Could you check a few things on this model? Use its own coordinates, in mm. Face numbers are marked on the shaded views. Coordinates: 2 decimals unless noted, no trailing zeros. Write each loop counter-clockwise with the first axis right and the second up, starting at its lowest first coordinate (ties: lowest second). Pieces come first, ordered by that corner, then holes. Notation, with made-up numbers: (10.5, 62.5) - (54.5, 62.5) arc R19 cw to (54.5, 69.5) - close; hole circle Ø4 at (50.5, -10.5). An arc over 180 degrees is marked (long way). Answer as a JSON object with one key per item and string values. Group by question number.
1) We'd pull the mould along X, two halves only. Please class the marked faces 1, 2 and 3: released by +X, released by -X, zero draft, split by the parting line, or undercut.
2) Will these pins go through, and if not, where does the flat tip stop? pin 1 Ø1.5 at (x, y) = (2, -4) entering from -Z; pin 2 Ø1.5 at (x, z) = (4, 0.5) entering from +Y; pin 3 Ø5 at (y, z) = (3.5, -1) entering from +X.
3) If we section it at D-D (z = 3.25): Write out the boundary of the cut face in (x, y), plus the area to 3 significant figures.
4) If we section it at C-C (z = -2.75): Write out the boundary of the cut face in (x, y).
5) If we section it at A-A (y = 0): Write out the boundary of the cut face in (x, z), plus the area to 3 significant figures.
6) If we section it at B-B (x = 0): Write out the boundary of the cut face in (y, z).
7) Please list where these lines run through material, in increasing order: line 1 along Y through (x, z) = (0, 5.3); line 2 along Z through (x, y) = (6.25, 0.25); line 3 along X through (y, z) = (3.5, 3.75).
```python
from build123d import *

# Parameters (mm, degrees)
SKETCH_1_R          = 6.9
EXTRUDE_1_DEPTH     = 6.8
SKETCH_2_R          = 0.35
EXTRUDE_2_DEPTH     = 4.5
SKETCH_3_R          = 1
CUT_EXTRUDE_1_DEPTH = 4.5


with BuildPart() as part:
    # Эскиз1 → Бобышка-Вытянуть1 (new body)
    with BuildSketch(Plane.XY):
        Circle(SKETCH_1_R)
    extrude(amount=EXTRUDE_1_DEPTH)

    # Эскиз2 → Бобышка-Вытянуть2 (add)
    with BuildSketch(Plane(origin=(0, 0, 0), x_dir=(-1, 0, 0), z_dir=(0, 0, -1))):
        with Locations(Location((0, 3.8, 0), (0, 0, 180))):
            Circle(SKETCH_2_R)
        with Locations(Location((0, -3.8, 0), (0, 0, 180))):
            Circle(SKETCH_2_R)
    extrude(amount=EXTRUDE_2_DEPTH)

    # Эскиз3 → Вырез-Вытянуть1 (cut)
    with BuildSketch(Plane.XY.offset(6.8)):
        Circle(SKETCH_3_R)
    extrude(amount=-CUT_EXTRUDE_1_DEPTH, mode=Mode.SUBTRACT)


solid = part.part
```
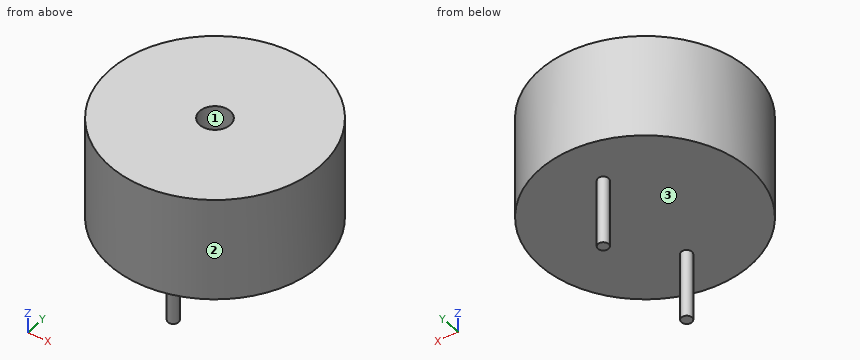
Here are the results:
{
 "1": {"face 1": "undercut", "face 2": "split by the parting line", "face 3": "zero draft"},
 "2": {"pin 1": "stops at z = 0", "pin 2": "stops at y = 6.09", "pin 3": "stops at x = 6.79"},
 "3": {"outline": "circle Ø13.8 at (0, 0); hole circle Ø2 at (0, 0)", "area": "146 mm²"},
 "4": {"outline": "circle Ø0.7 at (0, -3.8); circle Ø0.7 at (0, 3.8)"},
 "5": {"outline": "(-6.9, 0) - (6.9, 0) - (6.9, 6.8) - (1, 6.8) - (1, 2.3) - (-1, 2.3) - (-1, 6.8) - (-6.9, 6.8) - close", "area": "84.8 mm²"},
 "6": {"outline": "(-6.9, 0) - (-4.15, 0) - (-4.15, -4.5) - (-3.45, -4.5) - (-3.45, 0) - (3.45, 0) - (3.45, -4.5) - (4.15, -4.5) - (4.15, 0) - (6.9, 0) - (6.9, 6.8) - (1, 6.8) - (1, 2.3) - (-1, 2.3) - (-1, 6.8) - (-6.9, 6.8) - close"},
 "7": {"line 1": "y = -6.9 to -1, 1 to 6.9", "line 2": "z = 0 to 6.8", "line 3": "x = -5.95 to 5.95"}
}
